```python
from build123d import *

# Parameters (mm, degrees)
CORTAR_EXTRUIR1_DEPTH = 46.56245087


with BuildPart() as part:
    # Croquis2 → Revolución1 (revolve)
    with BuildSketch(Plane.XY, mode=Mode.PRIVATE) as revoluci_n1_sk:
        Polygon((0, -14.74724396), (3.75, -14.74724396), (3.75, -11.74724396), (2, -9.74724396), (2, 45.25275604), (0, 45.25275604), align=None)
    revolve(revoluci_n1_sk.sketch.rotate(Axis((0, 34.083509453, 0), (0, -1, 0)), 90), axis=Axis((0, 34.083509453, 0), (0, -1, 0)))

    # Croquis3 → Cortar-Extruir1 (cut, through all)
    with BuildSketch(Plane.XY):
        Polygon((2, 45.25275604), (2, 43.25275604), (1.015724773, 43.25275604), (1.015724773, 42.75275604), (2, 42.75275604), (2, 40.75275604), (1.015724773, 40.75275604), (1.015724773, 40.25275604), (2, 40.25275604), (2, 38.25275604), (1.015724773, 38.25275604), (1.015724773, 37.75275604), (2, 37.75275604), (2, 35.75275604), (1.015724773, 35.75275604), (1.015724773, 35.25275604), (2, 35.25275604), (2, 33.25275604), (1.015724773, 33.25275604), (1.015724773, 32.75275604), (2, 32.75275604), (2, 30.75275604), (1.015724773, 30.75275604), (1.015724773, 30.25275604), (2, 30.25275604), (2, 28.25275604), (1.015724773, 28.25275604), (1.015724773, 27.75275604), (2, 27.75275604), (2, 25.75275604), (1.015724773, 25.75275604), (1.015724773, 25.25275604), (2, 25.25275604), (2, 23.25275604), (1.015724773, 23.25275604), (1.015724773, 22.75275604), (2, 22.75275604), (2, 20.75275604), (1.015724773, 20.75275604), (1.015724773, 20.25275604), (2, 20.25275604), (3.93485594, 20.25275604), (3.93485594, 45.25275604), align=None)
    extrude(amount=-CORTAR_EXTRUIR1_DEPTH, mode=Mode.SUBTRACT)


solid = part.part
```
The listing builds one solid part. Answer for the finished solid, in the listing's coordinates (mm). A direction names the side the tool comes from. Coordinates: 2 decimals unless noted, no trailing zeros. Write each loop counter-clockwise with the first axis right and the second up, starting at its lowest first coordinate (ties: lowest second). Pieces come first, ordered by that corner, then holes. Notation, with made-up numbers: (27.5, 56) - (61.5, 56) arc R11 cw to (61.5, 69) - close; hole circle Ø11 at (45, -16). An arc over 180 degrees is marked (long way). One line per item, written item: value.
1) Each of these flat-tipped pins is pushed along its axis until it touches: pin 1 Ø2 at (y, z) = (32.5, -2.5) entering from +X; pin 2 Ø1 at (y, z) = (19.5, -1.5) entering from -X. Where does it stop, or does it pass through?
Geometry check:
pin 1: stops at x = 1.32
pin 2: stops at x = -1.73
2) Consider line 1 along X through (y, z) = (-1, -1); line 2 along X through (y, z) = (21, -0.25); line 3 along Y through (x, z) = (2.5, 2.75). Determine where each line is inside the solid, lowest interval first. Write a range as from..to.
Geometry check:
line 1: x = -1.73..1.73
line 2: x = -1.98..1.98
line 3: y = -14.75..-11.71
3) A tool of negligible diameter and unlimited length cuts with its end or side. For faces 4 (the cylindrical face through (-1.686, 18.138, 1.075)), 5 (the flat face through (1.4, 42.753, -0.7)), from which of +Z, -Z, +X, -X, +Y, -Y can it reach the whole face along a straight path? Write none if from no direction.
Geometry check:
face 4: +Y
face 5: -Z, +X
4) For a pull along Y with two mould halves and no side action, classify faces 1 (the flat face through (1.4, 22.753, -0.7)), 2 (the flat face through (0, 45.253, 0)), 3 (the flat face through (1.4, 35.253, -0.7)) as pulls with the +Y half, pulls with the -Y half, needs draft (parallel to the pull), parting line crosses it, or undercut.
Geometry check:
face 1: undercut
face 2: pulls with the +Y half
face 3: undercut
5) Find section A-A (y = 6). Give the vertices of the cut face in (x, z).
Geometry check:
outline: circle Ø4 at (0, 0)
